Geometry: final body of the model. Coordinates: model frame, mm. A direction names the side the tool comes from. Coordinates: 2 decimals unless noted, no trailing zeros. Order: outer loops, then holes, each group sorted by start corner. A loop starts at its lowest first (then second) coordinate and runs counter-clockwise, first axis right, second up. Notation, with made-up numbers: (87.5, -19) -> (128.5, -19) arc R17 cw to (128.5, 5) -> close; hole circle Ø5 at (15.5, -37). An arc over 180 degrees is marked (long way). Answer in a Markdown table with one row per item. Add a question column.
1) Section query D-D on x = 7.5. Return the cut outline in (y, z).
2) Set-up query: faces 1 (the face through (12.5, 5, 12)), 2 (the face through (-18.25, 0.08, -14.22)), 3 (the face through (20.1, -6.02, 12.91)), 4 (the face through (-20, 4, 16.25)). Return all of +Z, -Z, +X, -X, +Y, -Y with unobstructed straight access to the full face (end or side cutting, diameter ignored); none if empty.
3) Section query A-A on y = 0. Count the separate pieces of the cut face and the enclosed holes in it, then the cut area to 3 significant figures.
4) Section query C-C on y = 3.75. Return the cut outline in (x, z), then the cut area to 3 significant figures.
5) Ray query, line 1 (X direction, y = 0, z = 13.25); line 2 (Z direction, x = 17.75, y = 0); line 3 (Y direction, x = -20, z = 14.15). Return the intervals inside material, ascending. Write a range as from..to.
6) Pull-direction query (Z, two-part tool) for faces 5 (the face through (19.895, -4.765, -15.708)), 6 (the face through (20.105, -6.008, -12.885)), 7 (the face through (27.5, 11, 9)); classes: +Z half, -Z half, draft (parallel to the pull), parting line (faces both ways), or undercut.
7) Contact query for flat-ended pins moving along their axis: P1, Ø12, axis at x = 23, y = 8, coming from the +Z side; P2, Ø4.5, axis at x = -20, y = 0, coming from the -Z side; P3, Ø4.5, axis at x = 20, y = 0, coming from the +Z side; P4, Ø10, axis at x = 1, z = 29.5, coming from the -Y side. Output: stop coordinate, or through.
8) Section query B-B on x = -20. Return the cut outline in (y, z), then the cut area to 3 significant figures.
```python
from build123d import *

# Parameters (mm, degrees)
SKETCH_1_R               = 12.25
EXTRUDE_1_DEPTH          = 27.5
CUT_EXTRUDE_2_DEPTH      = 1
CUT_EXTRUDE_2_DEPTH_BACK = 56
EXTRUDE_2_DEPTH          = 55
FILLET_1_R               = 1
SKETCH_5_R               = 1.75
CUT_EXTRUDE_3_DEPTH      = 61
SKETCH_2_W               = 25
SKETCH_2_H               = 30
CUT_EXTRUDE_1_DEPTH      = 33.5000001
FILLET_2_R               = 10
CHAMFER_1_SIZE           = 3


with BuildPart() as part:
    # ｽｹｯﾁ1 → ﾎﾞｽ - 押し出し1 (new body, symmetric)
    with BuildSketch(Plane(origin=(0, 0, 0), x_dir=(0, 0, -1), z_dir=(1, 0, 0))):
        with BuildLine():
            Line((16.25, 0), (16.25, 17.25))
            Line((16.25, 17.25), (-43.75, 17.25))
            Line((-43.75, 17.25), (-43.75, 12.25))
            Line((-43.75, 12.25), (-16.25, 12.25))
            Line((-16.25, 12.25), (-16.25, 0))
            ThreePointArc((-16.25, 0), (0, -16.25), (16.25, 0))
        make_face()
        Circle(SKETCH_1_R, mode=Mode.SUBTRACT)
    extrude(amount=EXTRUDE_1_DEPTH, both=True)

    # ｽｹｯﾁ3 → ｶｯﾄ - 押し出し2 (cut, two sides)
    with BuildSketch(Plane(origin=(27.5, 0, 0), x_dir=(0, 0, -1), z_dir=(1, 0, 0))) as cut_extrude_2_sk:
        Polygon((-152.616304173, -71.166151395), (-17.557784777, -8.187329502), (0, 0), (20.401420048, -9.513338406), (155.459939444, -72.492160299), (154.177134941, -370.530575754), (-153.899108676, -369.20456685), align=None)
    extrude(amount=CUT_EXTRUDE_2_DEPTH, mode=Mode.SUBTRACT)
    extrude(cut_extrude_2_sk.sketch, amount=-CUT_EXTRUDE_2_DEPTH_BACK, mode=Mode.SUBTRACT)

    # ｽｹｯﾁ4 → ﾎﾞｽ - 押し出し2 (add)
    with BuildSketch(Plane.ZY.offset(27.5)):
        with BuildLine():
            Line((16.25, 0), (16.25, -3.602538268))
            Line((16.25, -3.602538268), (14.727501539, -6.867546753))
            ThreePointArc((14.727501539, -6.867546753), (15.864810116, -3.517143726), (16.25, 0))
        make_face()
        with BuildLine():
            Line((-16.25, 0), (-16.25, -3.602538268))
            Line((-16.25, -3.602538268), (-14.727501539, -6.867546753))
            ThreePointArc((-14.727501539, -6.867546753), (-15.864810116, -3.517143726), (-16.25, 0))
        make_face()
    extrude(amount=-EXTRUDE_2_DEPTH)

    # ﾌｨﾚｯﾄ1
    fillet_1_edges = [part.edges().sort_by_distance(p)[0] for p in [
        (0, -5.177073706, -11.102270391),
        (0, -5.177073706, 11.102270391),
        (0, -6.867546753, 14.727501539),
        (0, -6.867546753, -14.727501539),
    ]]
    fillet(fillet_1_edges, radius=FILLET_1_R)

    # ｽｹｯﾁ5 → ｶｯﾄ - 押し出し3 (cut, through all)
    with BuildSketch(Plane(origin=(0, 0, -16.25), x_dir=(-1, 0, 0), z_dir=(0, 0, -1))):
        with Locations((20, 0)):
            Circle(SKETCH_5_R)
        with Locations((-20, 0)):
            Circle(SKETCH_5_R)
    extrude(amount=-CUT_EXTRUDE_3_DEPTH, mode=Mode.SUBTRACT)

    # ｽｹｯﾁ2 → ｶｯﾄ - 押し出し1 (cut, through all)
    with BuildSketch(Plane.XY.offset(16.25)):
        with Locations((0, -2.75)):
            Rectangle(SKETCH_2_W, SKETCH_2_H)
    extrude(amount=-CUT_EXTRUDE_1_DEPTH, mode=Mode.SUBTRACT)

    # ﾌｨﾚｯﾄ2
    fillet_2_edges = [part.edges().sort_by_distance(p)[0] for p in [
        (27.5, 14.75, 43.75),
        (-27.5, 14.75, 43.75),
    ]]
    fillet(fillet_2_edges, radius=FILLET_2_R)

    # 面取り1
    chamfer_1_edges = [part.edges().sort_by_distance(p)[0] for p in [
        (0, 17.25, -16.25),
    ]]
    chamfer(chamfer_1_edges, length=CHAMFER_1_SIZE)


solid = part.part
```
Result:
| question | item | result |
|---|---|---|
| 1 | outline | (12.25, -16.25) -> (14.25, -16.25) -> (17.25, -13.25) -> (17.25, 43.75) -> (12.25, 43.75) -> close |
| 2 | face 1 | +Z, -Z, -Y |
| 2 | face 2 | +Z, -Z |
| 2 | face 3 | +X, -X, -Y |
| 2 | face 4 | +Z, +X, -X, -Y |
| 3 | separate pieces | 8 |
| 3 | enclosed holes | 0 |
| 3 | area | 184 mm2 |
| 4 | outline | (-27.5, -16.25) -> (-12.5, -16.25) -> (-12.5, -11.66) -> (-27.5, -11.66) -> close; (-27.5, 11.66) -> (-12.5, 11.66) -> (-12.5, 16.25) -> (-27.5, 16.25) -> close; (12.5, -16.25) -> (27.5, -16.25) -> (27.5, -11.66) -> (12.5, -11.66) -> close; (12.5, 11.66) -> (27.5, 11.66) -> (27.5, 16.25) -> (12.5, 16.25) -> close |
| 4 | area | 275 mm2 |
| 5 | line 1 | -27.5..-21.75, -18.25..-12.5, 12.5..18.25, 21.75..27.5 |
| 5 | line 2 | -16.25..-12.25, 12.25..16.25 |
| 5 | line 3 | -6.53..-1.75, 1.75..17.25 |
| 6 | face 5 | -Z half |
| 6 | face 6 | undercut |
| 6 | face 7 | draft |
| 7 | P1 | z = 43.67 |
| 7 | P2 | z = -16.25 |
| 7 | P3 | z = 16.25 |
| 7 | P4 | y = 12.25 |
| 8 | outline | (-6.44, -13.82) arc R1 ccw to (-5.96, -15.15) -> (-3.6, -16.25) -> (-1.75, -16.25) -> (-1.75, -12.12) arc R12.25 cw to (-4.32, -11.46) arc R1 ccw to (-5.58, -11.97) -> close; (-6.44, 13.82) -> (-5.58, 11.97) arc R1 ccw to (-4.32, 11.46) arc R12.25 cw to (-1.75, 12.12) -> (-1.75, 16.25) -> (-3.6, 16.25) -> (-5.96, 15.15) arc R1 ccw to start; (1.75, -16.25) -> (14.25, -16.25) -> (17.25, -13.25) -> (17.25, 43.43) -> (12.25, 43.43) -> (12.25, 16.25) -> (1.75, 16.25) -> (1.75, 12.12) arc R12.25 cw to (1.75, -12.12) -> close |
| 8 | area | 479 mm2 |
